The listing builds one solid part. Answer for the finished solid, in the listing's coordinates (mm). A direction names the side the tool comes from. Round coordinates to 2 decimals unless told otherwise and drop trailing zeros. Write each loop counter-clockwise with the first axis right and the second up, starting at its lowest first coordinate (ties: lowest second). Pieces come first, ordered by that corner, then holes. Notation, with made-up numbers: (42.25, 57) - (70.25, 57) arc R31 ccw to (70.25, 86) - close; hole circle Ø2 at (56.25, -11). An arc over 180 degrees is marked (long way). Answer in a Markdown table with one row per item.
Autodesk Inventor part; units mm, degrees
ref_plane "YZ Plane" through (0, 0, 0) normal (1, 0, 0) x (0, 1, 0)
ref_plane "XZ Plane" through (0, 0, 0) normal (0, 1, 0) x (-1, 0, 0)
ref_plane "XY Plane" through (0, 0, 0) normal (0, 0, 1) x (1, 0, 0)
sketch "Sketch1" plane through (0, 0, 0) normal (0, 1, 0) x (-1, 0, 0)
  line L0 (-12.7, 12.7) -> (12.7, 12.7)
  line L1 (12.7, 12.7) -> (12.7, -12.7)
  line L2 (12.7, -12.7) -> (-12.7, -12.7)
  line L3 (-12.7, -12.7) -> (-12.7, 12.7)
  line L4 (-12.7, 12.7) -> (12.7, -12.7) construction
  line L5 (12.7, 12.7) -> (-12.7, -12.7) construction
  line L6 (11.1125, -11.1125) -> (11.1125, 11.1125)
  line L7 (11.1125, 11.1125) -> (-11.1125, 11.1125)
  line L8 (-11.1125, 11.1125) -> (-11.1125, -11.1125)
  line L9 (-11.1125, -11.1125) -> (11.1125, -11.1125)
  point P0 (0, 0)
  dimension "d0" = 25.4
  dimension "d1" = 25.4
  dimension "d2" = 1.5875
extrude "Extrusion1" add sketch "Sketch1" along normal blind 220.98
sketch "Sketch2" plane through (12.7, 0, 12.7) normal (1, 0, 0) x (0, 0, -1)
  line L0 (12.7, 0) -> (22.225, 0) construction
  line L1 (0, 0) -> (25.4, 0) construction
  line L2 (12.7, 0) -> (3.175, 0) construction
  line L3 (3.175, 0) -> (3.175, 19.05) construction
  line L4 (3.175, 19.05) -> (22.225, 19.05) construction
  line L5 (22.225, 19.05) -> (22.225, 0) construction
  line L6 (3.175, 19.05) -> (22.225, 0) construction
  line L7 (22.225, 19.05) -> (3.175, 0) construction
  circle A0 centre (12.7, 9.525) radius 2.4384
  dimension "d5" = 9.525
  dimension "d7" = 9.525
  dimension "d8" = 19.05
  dimension "d9" = 4.8768
extrude "Extrusion2" cut sketch "Sketch2" against normal blind 25.4
sketch "Sketch3" plane through (12.7, 0, -12.7) normal (0, 0, -1) x (-1, 0, 0)
  line L0 (12.7, 0) -> (22.225, 0) construction
  line L1 (0, 0) -> (25.4, 0) construction
  line L2 (12.7, 0) -> (3.175, 0) construction
  line L3 (3.175, 0) -> (3.175, 19.05) construction
  line L4 (3.175, 19.05) -> (22.225, 19.05) construction
  line L5 (22.225, 19.05) -> (22.225, 0) construction
  line L6 (3.175, 19.05) -> (22.225, 0) construction
  line L7 (22.225, 19.05) -> (3.175, 0) construction
  circle A0 centre (12.7, 9.525) radius 2.4384
  point P0 (12.7, 0)
  dimension "d13" = 9.525
  dimension "d14" = 9.525
  dimension "d15" = 19.05
  dimension "d16" = 4.8768
extrude "Extrusion3" cut sketch "Sketch3" against normal blind 25.4
sketch "Sketch4" plane through (12.7, 0, 12.7) normal (1, 0, 0) x (0, 0, -1)
  circle A0 centre (12.7, 208.28) radius 2.4384
  circle A1 centre (12.7, 182.88) radius 2.4384
  line L0 (0, 220.98) -> (25.4, 220.98)
  point P0 (12.7, 0)
  dimension "d19" = 12.7
  dimension "d20" = 4.8768
  dimension "d21" = 25.4
extrude "Extrusion4" cut sketch "Sketch4" against normal blind 7.62
equation "\"d7\" = d5"
equation "\"d14\" = d13"
properties part number "metal tube piece"
(1) For a pull along Y with two mould halves and no side action, classify faces 1 (the flat face through (0, 109, 11.112)), 2 (the flat face through (11.3, 220.98, 0.1)), 3 (the cylindrical face through (11.917, 11.943, 0.317)), 4 (the cylindrical face through (-11.895, 11.943, 0.317)) as pulls with the +Y half, pulls with the -Y half, needs draft (parallel to the pull), parting line crosses it, or undercut.
Checked values:
| item | result |
|---|---|
| face 1 | needs draft |
| face 2 | pulls with the +Y half |
| face 3 | undercut |
| face 4 | undercut |
(2) Section B-B (z = 0) is taken. Give the vertices of the cut face in (x, y).
Checked values:
| item | result |
|---|---|
| outline | (-12.7, 0) - (-11.11, 0) - (-11.11, 7.09) - (-12.7, 7.09) - close; (-12.7, 11.96) - (-11.11, 11.96) - (-11.11, 220.98) - (-12.7, 220.98) - close; (11.11, 0) - (12.7, 0) - (12.7, 7.09) - (11.11, 7.09) - close; (11.11, 11.96) - (12.7, 11.96) - (12.7, 180.44) - (11.11, 180.44) - close; (11.11, 185.32) - (12.7, 185.32) - (12.7, 205.84) - (11.11, 205.84) - close; (11.11, 210.72) - (12.7, 210.72) - (12.7, 220.98) - (11.11, 220.98) - close |
(3) Section D-D (z = 8.75) is taken. Give the vertices of the cut face in (x, y), and give its area (3 significant figures).
Checked values:
| item | result |
|---|---|
| outline | (-12.7, 0) - (-11.11, 0) - (-11.11, 220.98) - (-12.7, 220.98) - close; (11.11, 0) - (12.7, 0) - (12.7, 220.98) - (11.11, 220.98) - close |
| area | 702 mm2 |
(4) Section C-C (y = 67) is taken. Give the vertices of the cut face in (x, z), and give its area (3 significant figures).
Checked values:
| item | result |
|---|---|
| outline | (-12.7, -12.7) - (12.7, -12.7) - (12.7, 12.7) - (-12.7, 12.7) - close; hole (-11.11, -11.11) - (11.11, -11.11) - (11.11, 11.11) - (-11.11, 11.11) - close |
| area | 151 mm2 |
(5) Section A-A (x = 0) is taken. Give the vertices of the cut face in (y, z), and give its area (3 significant figures).
Checked values:
| item | result |
|---|---|
| outline | (0, -12.7) - (7.09, -12.7) - (7.09, -11.11) - (0, -11.11) - close; (0, 11.11) - (7.09, 11.11) - (7.09, 12.7) - (0, 12.7) - close; (11.96, -12.7) - (220.98, -12.7) - (220.98, -11.11) - (11.96, -11.11) - close; (11.96, 11.11) - (220.98, 11.11) - (220.98, 12.7) - (11.96, 12.7) - close |
| area | 686 mm2 |
(6) Find the intervals of material crossed by line 1 (Y direction, x = 12, z = 0); line 2 (X direction, y = 75, z = 1.75), in increasing order.
Checked values:
| item | result |
|---|---|
| line 1 | y = 0 to 7.09, 11.96 to 180.44, 185.32 to 205.84, 210.72 to 220.98 |
| line 2 | x = -12.7 to -11.11, 11.11 to 12.7 |
(7) For faces 5 (the cylindrical face through (11.9, 210.7, 0.3)), 6 (the flat face through (-11.112, 109, 0)), 7 (the flat face through (11.3, 0, 0.1)), determine the directions among +Z, -Z, +X, -X, +Y, -Y from which every point of the face is accessible in a straight line to the end or side of a thin tool.
Checked values:
| item | result |
|---|---|
| face 5 | +X |
| face 6 | +Y, -Y |
| face 7 | +Z, -Z, +X, -X, -Y |
